Here's the drawing with two shaded views (mm, measured from the low corner). I have some questions. A direction names the side the tool comes from. Coordinates: 2 decimals unless noted, no trailing zeros. Loops run counter-clockwise (first coordinate to the right, second up) from the corner with the lowest first, then second, coordinate; pieces in that order, holes last.
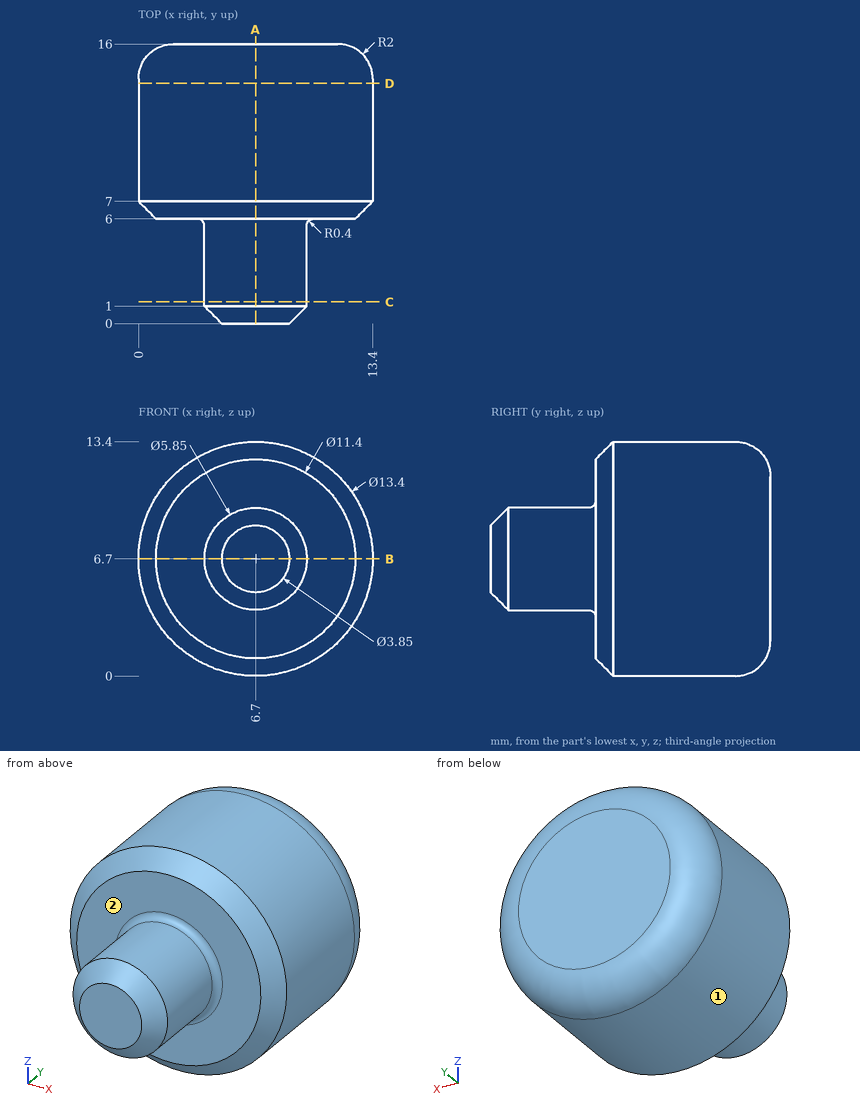
(1) Which directions (+Z, -Z, +X, -X, +Y, -Y) give clear straight access to the entire face, cutting with the end or side of a thin tool? Please do the marked faces 1 and 2.
Check values:
face 1: +Y, -Y
face 2: -Y
(2) I'm going to push flat-ended pins straight in: pin 1 (5 mm diameter, centred on y = 5.5, z = 2, fed in from -X); pin 2 (4 mm diameter, centred on y = 11, z = 12, fed in from +X); pin 3 (1 mm diameter, centred on y = 12.5, z = 5.5, fed in from -X). Where does each tip first touch, or does it pass through?
Check values:
pin 1: stops at x = 0.57
pin 2: stops at x = 12.53
pin 3: stops at x = 0.04
(3) I want a section at C-C on y = 1.25. Write out the boundary of the cut face in (x, z) (3 decimals).
Check values:
outline: circle Ø5.85 at (6.7, 6.7)
(4) If I drill on probe 1 along Y at (x, z) = (9.5, 8.75); probe 2 along Z at (x, y) = (6.5, 13); probe 3 along X at (y, z) = (15.25, 12), over which ranges is the centre line in solid material (lowest first)?
Check values:
probe 1: y = 6 to 16
probe 2: z = 0 to 13.4
probe 3: x = 3.37 to 10.03
(5) I want a section at B-B on z = 6.7. Write out the boundary of the cut face in (x, y) (3 decimals), then the cut area to 3 significant figures.
Check values:
outline: (0, 7) - (1, 6) - (3.375, 6) arc R0.4 cw to (3.775, 5.6) - (3.775, 1) - (4.775, 0) - (8.625, 0) - (9.625, 1) - (9.625, 5.6) arc R0.4 cw to (10.025, 6) - (12.4, 6) - (13.4, 7) - (13.4, 14) arc R2 ccw to (11.4, 16) - (2, 16) arc R2 ccw to (0, 14) - close
area: 165 mm2
(6) I want a section at D-D on y = 13.75. Write out the boundary of the cut face in (x, z).
Check values:
outline: circle Ø13.4 at (6.7, 6.7)
(7) I want a section at A-A on x = 6.7. Write out the boundary of the cut face in (y, z) (3 decimals), then the cut area to 3 significant figures.
Check values:
outline: (0, 4.775) - (1, 3.775) - (5.6, 3.775) arc R0.4 cw to (6, 3.375) - (6, 1) - (7, 0) - (14, 0) arc R2 ccw to (16, 2) - (16, 11.4) arc R2 ccw to (14, 13.4) - (7, 13.4) - (6, 12.4) - (6, 10.025) arc R0.4 cw to (5.6, 9.625) - (1, 9.625) - (0, 8.625) - close
area: 165 mm2
